from build123d import *

# Parameters (mm, degrees)
SKETCH1_R           = 40
BOSS_EXTRUDE1_DEPTH = 2
SKETCH5_R           = 1.5
CUT_EXTRUDE2_DEPTH  = 3
SKETCH7_R           = 1
CUT_EXTRUDE4_DEPTH  = 3
SKETCH8_R           = 30.471270003
CUT_EXTRUDE5_DEPTH  = 3
CIRPATTERN1_COUNT   = 3
FILLET1_R           = 2


with BuildPart() as part:
    # Sketch1 → Boss-Extrude1 (new body)
    with BuildSketch(Plane(origin=(0, 0, 0), x_dir=(1, 0, 0), z_dir=(0, 1, 0))):
        Circle(SKETCH1_R)
    extrude(amount=BOSS_EXTRUDE1_DEPTH)

    # Sketch5 → Cut-Extrude2 (cut, through all)
    with BuildSketch(Plane(origin=(0, 2, 0), x_dir=(1, 0, 0), z_dir=(0, 1, 0))):
        with Locations((0, 36)):
            Circle(SKETCH5_R)
    extrude(amount=-CUT_EXTRUDE2_DEPTH, mode=Mode.SUBTRACT)

    # Sketch7 → Cut-Extrude4 (cut, through all)
    with BuildSketch(Plane(origin=(0, 2, 0), x_dir=(1, 0, 0), z_dir=(0, 1, 0))):
        Circle(SKETCH7_R)
    extrude(amount=-CUT_EXTRUDE4_DEPTH, mode=Mode.SUBTRACT)

    # Sketch8 → Cut-Extrude5 (cut, through all)
    with BuildSketch(Plane(origin=(0, 2, 0), x_dir=(1, 0, 0), z_dir=(0, 1, 0))):
        with Locations((40.698571494, 23.497331208)):
            Circle(SKETCH8_R)
    cut_extrude5 = extrude(amount=-CUT_EXTRUDE5_DEPTH, mode=Mode.SUBTRACT)

    # CirPattern1: Cut-Extrude5 ×3 about axis
    cirpattern1_axis = Axis((0, 0, 0), (0, 1, 0))
    for i in range(1, CIRPATTERN1_COUNT):
        add(cut_extrude5.rotate(cirpattern1_axis, i * 360 / CIRPATTERN1_COUNT), mode=Mode.SUBTRACT)

    # Fillet1
    fillet1_edges = [part.edges().sort_by_distance(p)[0] for p in [
        (39.39231012, 1, 6.945927107),
        (13.680805733, 1, -37.587704831),
        (-25.711504387, 1, 30.641777725),
        (25.711504387, 1, 30.641777725),
        (-13.680805733, 1, -37.587704831),
        (-39.39231012, 1, 6.945927107),
    ]]
    fillet(fillet1_edges, radius=FILLET1_R)


solid = part.part
Work out the finished part from the listing and answer in its coordinate system (mm). Give positions to 0.01 mm unless a question says otherwise; leave off trailing zeros. Order: outer loops, then holes, each group sorted by start corner. A loop starts at its lowest first (then second) coordinate and runs counter-clockwise, first axis right, second up. Notation, with made-up numbers: (45, 77) -> (60, 77) arc R20 ccw to (60, 84) -> close; hole circle Ø2 at (46.5, 14.25). An arc over 180 degrees is marked (long way). One line per item, written item: value.
Item 1: Find section B-B, the plane x = 0. Give the vertices of the cut face in (y, z), plus the area to 3 significant figures.
Answer sheet:
outline: (0, -40) -> (2, -40) -> (2, -37.5) -> (0, -37.5) -> close; (0, -34.5) -> (2, -34.5) -> (2, -1) -> (0, -1) -> close; (0, 1) -> (2, 1) -> (2, 16.52) -> (0, 16.52) -> close
area: 103 mm²
Item 2: Straight lines are drawn through the part: probe 1 along Z at (x, y) = (0, 0.4); probe 2 along X at (y, z) = (1.5, -36); probe 3 along X at (y, z) = (0.5, 0). For each, find the intervals that lie inside material, in ascending order.
Answer sheet:
probe 1: -40 to -37.5, -34.5 to -1, 1 to 16.52
probe 2: -12.86 to -1.5, 1.5 to 12.86
probe 3: -21.3 to -1, 1 to 21.3
Item 3: Find section A-A, the plane z = 0. Give the vertices of the cut face in (x, y).
Answer sheet:
outline: (-21.3, 0) -> (-1, 0) -> (-1, 2) -> (-21.3, 2) -> close; (1, 0) -> (21.3, 0) -> (21.3, 2) -> (1, 2) -> close
Item 4: Find section D-D, the plane z = 18.5. Give the vertices of the cut face in (x, y).
Answer sheet:
outline: (-35.46, 0) -> (-10.8, 0) -> (-10.8, 2) -> (-35.46, 2) -> close; (10.8, 0) -> (35.46, 0) -> (35.46, 2) -> (10.8, 2) -> close
Item 5: Determine the mould class of faces 1 (the flat face through (-1, 0, 2)), 2 (the cylindrical face through (-34.7, 1, 19.9)), 3 (the cylindrical face through (-0.325, 1.014, -34.536)), 4 (the cylindrical face through (14.11, 1.01, -8.61)) for opening direction Z: released by +Z, released by -Z, zero draft, split by the parting line, or undercut.
Answer sheet:
face 1: zero draft
face 2: released by +Z
face 3: undercut
face 4: undercut
Item 6: A flat-ended cylindrical pin translates along its axis: P1, Ø1, axis at y = 0.5, z = 12.5, coming from the -X side. Find the tip coordinate at first contact, or state that the pin passes through.
Answer sheet:
P1: x = -38.16
Item 7: Find section C-C, the plane x = -33.5. Give the vertices of the cut face in (y, z), plus the area to 3 significant figures.
Answer sheet:
outline: (0, 6.11) -> (2, 6.11) -> (2, 21.86) -> (0, 21.86) -> close
area: 31.5 mm²
